```python
from build123d import *

# Parameters (mm, degrees)
SKETCH_1_R          = 31.26
EXTRUDE_1_DEPTH     = 16
SKETCH_2_R          = 5
CUT_EXTRUDE_1_DEPTH = 16
EXTRUDE_START       = 2
SKETCH_3_R          = 35.5
SKETCH_3_R_2        = 5
EXTRUDE_2_DEPTH     = 2
SKETCH_4_R          = 35.5
SKETCH_4_R_2        = 5
EXTRUDE_3_DEPTH     = 2


with BuildPart() as part:
    # 草图1 → 凸台-拉伸1 (new body)
    with BuildSketch(Plane.XY):
        Circle(SKETCH_1_R)
    extrude(amount=EXTRUDE_1_DEPTH)

    # 草图2 → 切除-拉伸1 (cut)
    with BuildSketch(Plane.XY.offset(16)):
        Circle(SKETCH_2_R)
    extrude(amount=-CUT_EXTRUDE_1_DEPTH, mode=Mode.SUBTRACT)

    # 草图3 → 凸台-拉伸2 (add)
    with BuildSketch(Plane.XY.offset(16).offset(EXTRUDE_START)):
        Circle(SKETCH_3_R)
        Circle(SKETCH_3_R_2, mode=Mode.SUBTRACT)
    extrude(amount=-EXTRUDE_2_DEPTH)

    # 草图4 → 凸台-拉伸3 (add)
    with BuildSketch(Plane(origin=(0, 0, 0), x_dir=(-1, 0, 0), z_dir=(0, 0, -1))):
        with Locations(Location((0, 0, 0), (0, 0, 180))):
            Circle(SKETCH_4_R)
        with Locations(Location((0, 0, 0), (0, 0, 180))):
            Circle(SKETCH_4_R_2, mode=Mode.SUBTRACT)
    extrude(amount=EXTRUDE_3_DEPTH)


solid = part.part
```
Could you check a few things on this model? Use its own coordinates, in mm. A direction names the side the tool comes from. Round coordinates to 2 decimals unless told otherwise and drop trailing zeros. Loops run counter-clockwise (first coordinate to the right, second up) from the corner with the lowest first, then second, coordinate; pieces in that order, holes last.
Q1. Please list where these lines run through material, in increasing order: L1, parallel to Z at x = 3, y = 31.5; L2, parallel to Y at x = 0, z = 3.75; L3, parallel to Y at x = 2, z = 7.5.
Q2. For P1, Ø12, axis at y = 19, z = 0, coming from the +X side; P2, Ø5, axis at x = -10, z = 3.5, coming from the +Y side; P3, Ø10, axis at x = 23.5, z = 5.5, coming from the -Y side; P4, Ø9, axis at x = 0, y = 0, coming from the -Z side, each with a flat end and sliding along its axis, tell me the tip position at first contact or that it passes through.
Q3. Thinking about a two-plate mould opening in X: for faces 3 (the flat face through (2.5, 31.4, 0)), 4 (the cylindrical face through (-7.696, 34.656, -0.986)), 5 (the cylindrical face through (-5, 0, 8)), which applies, pulls with the +X half, pulls with the -X half, needs draft (parallel to the pull), parting line crosses it, or undercut?
Q4. I want a section at A-A (y = 0). Write out the boundary of the cut face in (x, z), and give its area (3 significant figures).
Q5. I want a section at C-C (z = 10). Write out the boundary of the cut face in (x, y).
Q6. I want a section at D-D (x = 11.5). Write out the boundary of the cut face in (y, z).
Q7. On a 3-axis mill with a long thin cutter (end or side, diameter ignored), from which of +Z, -Z, +X, -X, +Y, -Y can I reach the whole of each face in a straight line? I mean faces 1 (the cylindrical face through (-7.696, -34.656, 17.014)), 2 (the flat face through (2.5, -31.4, 16)). Say none if no direction works.
Answer below:
1. L1: z = -2 to 0, 16 to 18
1. L2: y = -31.26 to -5, 5 to 31.26
1. L3: y = -31.2 to -4.58, 4.58 to 31.2
2. P1: stops at x = 33.03
2. P2: stops at y = 30.35
2. P3: stops at y = -25.2
2. P4: passes through
3. face 3: needs draft
3. face 4: parting line crosses it
3. face 5: undercut
4. outline: (-35.5, -2) - (-5, -2) - (-5, 18) - (-35.5, 18) - (-35.5, 16) - (-31.26, 16) - (-31.26, 0) - (-35.5, 0) - close; (5, -2) - (35.5, -2) - (35.5, 0) - (31.26, 0) - (31.26, 16) - (35.5, 16) - (35.5, 18) - (5, 18) - close
4. area: 1,080 mm2
5. outline: circle Ø62.52 at (0, 0); hole circle Ø10 at (0, 0)
6. outline: (-33.59, -2) - (33.59, -2) - (33.59, 0) - (29.07, 0) - (29.07, 16) - (33.59, 16) - (33.59, 18) - (-33.59, 18) - (-33.59, 16) - (-29.07, 16) - (-29.07, 0) - (-33.59, 0) - close
7. face 1: +Z, -Z
7. face 2: none
